Could you check a few things on this model? Use its own coordinates, in mm. Face numbers are marked on the shaded views. A direction names the side the tool comes from. Give positions to 0.01 mm unless a question says otherwise; leave off trailing zeros. Order: outer loops, then holes, each group sorted by start corner. A loop starts at its lowest first (then second) coordinate and runs counter-clockwise, first axis right, second up.
Autodesk Inventor part; units mm, degrees
ref_plane "YZ Plane" through (0, 0, 0) normal (1, 0, 0) x (0, 1, 0)
ref_plane "XZ Plane" through (0, 0, 0) normal (0, 1, 0) x (-1, 0, 0)
ref_plane "XY Plane" through (0, 0, 0) normal (0, 0, 1) x (1, 0, 0)
sketch "Sketch1" plane through (0, 0, 0) normal (0, 0, 1) x (1, 0, 0)
  line L0 (0, 0) -> (60, 0)
  line L1 (60, 0) -> (60, -30)
  line L2 (60, -30) -> (0, -30)
  line L3 (0, -30) -> (0, 0)
  dimension "d0" = 60
  dimension "d1" = 30
extrude "Extrusion1" add sketch "Sketch1" along normal blind 68
sketch "Sketch2" plane through (0, 0, 68) normal (0, 0, 1) x (1, 0, 0)
  circle A0 centre (15, -15) radius 5
  line L0 (0, -30) -> (60, -30)
  line L1 (0, 0) -> (0, -30)
  dimension "d4" = 10
  dimension "d5" = 15
  dimension "d6" = 15
extrude "Extrusion2" cut sketch "Sketch2" against normal blind 68
sketch "Sketch3" plane through (60, -30, 0) normal (1, 0, 0) x (0, 0, -1)
  line L0 (-60, 5) -> (-8, 5)
  line L1 (-8, 5) -> (-8, 25)
  line L2 (-8, 25) -> (-60, 25)
  line L3 (-60, 25) -> (-60, 5)
  line L4 (-60, 5) -> (-8, 25) construction
  line L5 (-8, 5) -> (-60, 25) construction
  line L6 (-68, 0) -> (-68, 30)
  line L7 (0, 0) -> (-68, 0)
  point P0 (0, 30)
  point P1 (-34, 15)
  dimension "d9" = 52
  dimension "d10" = 20
  dimension "d11" = 34
  dimension "d12" = 15
extrude "Extrusion3" cut sketch "Sketch3" against normal blind 52
full round fillet "Full Round Fillet1" first side at (42.6667, -5, 25.3333) centre faces at (8, -11.6667, 42.6667) second side at (42.6667, -25, 42.6667)
fillet "Fillet1" radius 15 2 edges at (0, 0, 34) (0, -30, 34)
properties part number "1st arm"
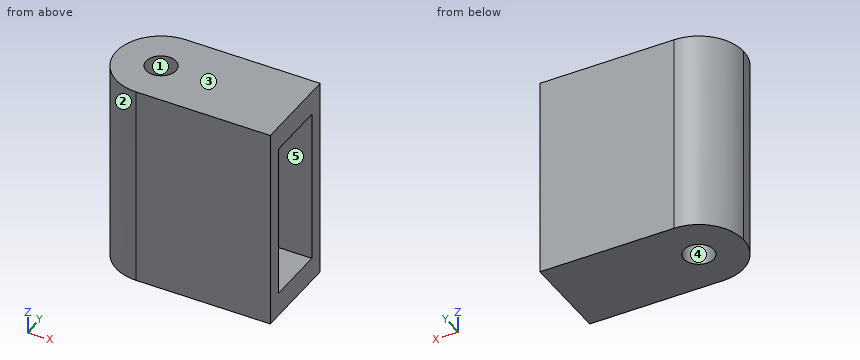
Item 1: For the marked faces 4 and 5, which set-ups out of +Z, -Z, +X, -X, +Y, -Y let a thin tool reach every point of the face, with its end or its side?
Findings:
face 4: +Z, -Z
face 5: +X
Item 2: Imagine slicing it at A-A on x = 49.5. List the corners of the cut face in (y, z) for me.
Findings:
outline: (-30, 0) - (0, 0) - (0, 68) - (-30, 68) - close; hole (-25, 8) - (-5, 8) - (-5, 60) - (-25, 60) - close
Item 3: Please list where these lines run through material, in increasing order: line 1 along Y through (x, z) = (34, 9.5); line 2 along Z through (x, y) = (42.5, -15.5); line 3 along Y through (x, z) = (15, 2).
Findings:
line 1: y = -30 to -25, -5 to 0
line 2: z = 0 to 8, 60 to 68
line 3: y = -30 to -20, -10 to 0
Item 4: For pin 1 (6 mm diameter, centred on x = 24.5, y = -6.5, fed in from -Z); pin 2 (1 mm diameter, centred on y = -25, z = 30, fed in from -X); pin 3 (5 mm diameter, centred on y = -13, z = 33.5, fed in from +X), each with a flat end and sliding along its axis, tell me the tip position at first contact or that it passes through.
Findings:
pin 1: stops at z = 0
pin 2: stops at x = 3.39
pin 3: stops at x = 9.07
Item 5: We'd pull the mould along Y, two halves only. Please class the marked faces 1, 2 and 3: +Y half, -Y half, draft (parallel to the pull), parting line (faces both ways), or undercut.
Findings:
face 1: undercut
face 2: -Y half
face 3: draft
Item 6: Imagine slicing it at B-B on y = -11.25. List the corners of the cut face in (x, z) for me, then the cut area to 3 significant figures.
Findings:
outline: (0.48, 0) - (11.69, 0) - (11.69, 8) - (8.73, 8) - (8.73, 60) - (11.69, 60) - (11.69, 68) - (0.48, 68) - close; (18.31, 0) - (60, 0) - (60, 8) - (18.31, 8) - close; (18.31, 60) - (60, 60) - (60, 68) - (18.31, 68) - close
area: 1,280 mm2
